Design review of the part built by this model. Coordinates are the model's own, in mm. A direction names the side the tool comes from. Give positions to 0.01 mm unless a question says otherwise; leave off trailing zeros. Order: outer loops, then holes, each group sorted by start corner. A loop starts at its lowest first (then second) coordinate and runs counter-clockwise, first axis right, second up. Notation, with made-up numbers: (59.5, 5) -> (80.5, 5) arc R24 ccw to (80.5, 38) -> close; hole circle Ø5 at (75.25, 57.25). An arc over 180 degrees is marked (long way). Answer in a Markdown table with one row per item. Add a question column.
```python
from build123d import *

# Parameters (mm, degrees)
ESQUISSE1_W              = 140
ESQUISSE1_H              = 30
BOSS_EXTRU_1_DEPTH       = 20
ESQUISSE3_W              = 140
ESQUISSE3_H              = 30
BOSS_EXTRU_2_DEPTH       = 20
BOSS_EXTRU_3_DEPTH       = 30
BOSS_EXTRU_4_DEPTH       = 30
ESQUISSE12_W             = 140
ESQUISSE12_H             = 30
ENL_V_MAT_EXTRU_1_DEPTH  = 41
ESQUISSE13_R             = 2
ENL_V_MAT_EXTRU_2_DEPTH  = 31
ESQUISSE25_R             = 2.5
ENL_V_MAT_EXTRU_11_DEPTH = 3
ENL_V_MAT_EXTRU_5_DEPTH  = 31
ENL_V_MAT_EXTRU_6_DEPTH  = 31
ESQUISSE19_W             = 12.781453569
ESQUISSE19_H             = 30
ENL_V_MAT_EXTRU_7_DEPTH  = 2
ESQUISSE20_W             = 12.289859201
ESQUISSE20_H             = 30
ENL_V_MAT_EXTRU_8_DEPTH  = 2
ENL_V_MAT_EXTRU_9_DEPTH  = 0.5
ENL_V_MAT_EXTRU_10_DEPTH = 0.5
ESQUISSE15_R             = 2.5
ENL_V_MAT_EXTRU_15_DEPTH = 3
CONG_1_R                 = 20
CONG_3_R                 = 4


with BuildPart() as part:
    # Esquisse1 → Boss.-Extru.1 (new body)
    with BuildSketch(Plane.XY):
        with Locations((70, 15)):
            Rectangle(ESQUISSE1_W, ESQUISSE1_H)
    extrude(amount=BOSS_EXTRU_1_DEPTH)

    # Esquisse3 → Boss.-Extru.2 (add)
    with BuildSketch(Plane.XY.offset(20)):
        with Locations((70, 15)):
            Rectangle(ESQUISSE3_W, ESQUISSE3_H)
    extrude(amount=BOSS_EXTRU_2_DEPTH)

    # Esquisse5 → Boss.-Extru.3 (add)
    with BuildSketch(Plane.XZ):
        Polygon((70, 12), (140, 25), (140, 12), (70, 0), align=None)
    extrude(amount=BOSS_EXTRU_3_DEPTH)

    # Esquisse6 → Boss.-Extru.4 (add)
    with BuildSketch(Plane.XZ):
        Polygon((0, 25), (0, 12.5), (70, 0), (70, 12), align=None)
    extrude(amount=BOSS_EXTRU_4_DEPTH)

    # Esquisse12 → Enlèv. mat.-Extru.1 (cut, through all)
    with BuildSketch(Plane.XY.offset(40)):
        with Locations((70, 15)):
            Rectangle(ESQUISSE12_W, ESQUISSE12_H)
    extrude(amount=-ENL_V_MAT_EXTRU_1_DEPTH, mode=Mode.SUBTRACT)

    # Esquisse13 → Enlèv. mat.-Extru.2 (cut, through all)
    with BuildSketch(Plane.XZ.offset(30)):
        with Locations((70, 6)):
            Circle(ESQUISSE13_R)
    extrude(amount=-ENL_V_MAT_EXTRU_2_DEPTH, mode=Mode.SUBTRACT)

    # Esquisse25 → Enlèv. mat.-Extru.11 (cut)
    with BuildSketch(Plane(origin=(2.1631644, 0, 12.113720643), x_dir=(-0.984427576, 0, 0.175790638), z_dir=(-0.175790638, 0, -0.984427576))):
        with Locations((-12.309930286, -15)):
            Circle(ESQUISSE25_R)
    extrude(amount=-ENL_V_MAT_EXTRU_11_DEPTH, mode=Mode.SUBTRACT)

    # Esquisse16 → Enlèv. mat.-Extru.5 (cut, through all)
    with BuildSketch(Plane(origin=(0, 0, 0), x_dir=(1, 0, 0), z_dir=(0, 1, 0))):
        Polygon((0, -12.5), (2.244032354, -24.583251134), (0, -25), align=None)
    extrude(amount=-ENL_V_MAT_EXTRU_5_DEPTH, mode=Mode.SUBTRACT)

    # Esquisse17 → Enlèv. mat.-Extru.6 (cut, through all)
    with BuildSketch(Plane(origin=(0, 0, 0), x_dir=(1, 0, 0), z_dir=(0, 1, 0))):
        Polygon((140, -12), (137.666206352, -24.56658118), (140, -25), align=None)
    extrude(amount=-ENL_V_MAT_EXTRU_6_DEPTH, mode=Mode.SUBTRACT)

    # Esquisse19 → Enlèv. mat.-Extru.7 (cut)
    with BuildSketch(Plane(origin=(137.486683764, 0, 25.53324127), x_dir=(0.182592194, 0, -0.983188736), z_dir=(0.983188736, 0, 0.182592194))):
        with Locations((7.373915521, -15)):
            Rectangle(ESQUISSE19_W, ESQUISSE19_H)
    extrude(amount=-ENL_V_MAT_EXTRU_7_DEPTH, mode=Mode.SUBTRACT)

    # Esquisse20 → Enlèv. mat.-Extru.8 (cut)
    with BuildSketch(Plane(origin=(-2.244032354, 0, 0.416748866), x_dir=(0.182592194, 0, 0.983188736), z_dir=(-0.983188736, 0, 0.182592194))):
        with Locations((18.434788802, -15)):
            Rectangle(ESQUISSE20_W, ESQUISSE20_H)
    extrude(amount=-ENL_V_MAT_EXTRU_8_DEPTH, mode=Mode.SUBTRACT)

    # Esquisse22 → Enlèv. mat.-Extru.9 (cut)
    with BuildSketch(Plane.XZ.offset(30)):
        Polygon((4.210409826, 24.218066747), (1.968902204, 12.148410321), (70, 0), (138.028566573, 11.662039984), (135.69982888, 24.201396792), (70, 12), align=None)
    extrude(amount=-ENL_V_MAT_EXTRU_9_DEPTH, mode=Mode.SUBTRACT)

    # Esquisse23 → Enlèv. mat.-Extru.10 (cut)
    with BuildSketch(Plane(origin=(0, 0, 0), x_dir=(1, 0, 0), z_dir=(0, 1, 0))):
        Polygon((1.968902204, -12.148410321), (4.210409826, -24.218066747), (70, -12), (135.69982888, -24.201396792), (138.028566573, -11.662039984), (70, 0), align=None)
    extrude(amount=-ENL_V_MAT_EXTRU_10_DEPTH, mode=Mode.SUBTRACT)

    # Esquisse15 → Enlèv. mat.-Extru.15 (cut)
    with BuildSketch(Plane(origin=(1.998413957, 0, -11.65741475), x_dir=(-0.985622255, 0, -0.168963815), z_dir=(0.168963815, 0, -0.985622255))):
        with Locations((-125.593557837, -15)):
            Circle(ESQUISSE15_R)
    extrude(amount=-ENL_V_MAT_EXTRU_15_DEPTH, mode=Mode.SUBTRACT)

    # Congé1
    cong_1_edges = [part.edges().sort_by_distance(p)[0] for p in [
        (70, -15, 12),
    ]]
    fillet(cong_1_edges, radius=CONG_1_R)

    # Congé3
    cong_3_edges = [part.edges().sort_by_distance(p)[0] for p in [
        (4.210409826, -15, 24.218066747),
        (104.675836379, -29.5, 18.439798185),
        (135.69982888, -15, 24.201396792),
        (35.279282974, -0.5, 18.448133162),
        (35.279282974, -29.5, 18.448133162),
        (104.675836379, -0.5, 18.439798185),
        (70, -0.5, 12.341974299),
        (70, -29.5, 12.341974299),
    ]]
    fillet(cong_3_edges, radius=CONG_3_R)


solid = part.part
```
1) For L1, parallel to Z at x = 70, y = -19.5; L2, parallel to Z at x = 25, y = -25.75; L3, parallel to Z at x = 75, y = -20.5, list the stretches that pass through material, from the lowest coordinate up.
2) Clearance check with flat-ended pins moving along their axes: P1, Ø3, axis at y = -5, z = 13, coming from the -X side; P2, Ø6, axis at y = -7.5, z = 19, coming from the +X side; P3, Ø4, axis at x = 25, y = -17, coming from the +Z side; P4, Ø12, axis at x = 32, y = -4, coming from the -Z side. State where each tip first meets the part, or that it passes through.
3) Machinability: for faces 1 (the face through (71.908, -15.203, 6.601)), 2 (the face through (34.636, -28.297, 17.407)), 3 (the face through (125.314, -14.965, 12.526)), 4 (the face through (37.7, -14.9, 18)), 5 (the face through (35.495, -1.641, 17.185)), which of the approach directions +Z, -Z, +X, -X, +Y, -Y give a long, thin tool a straight path to every point of the face, cutting with its end or side? Answer none if there is none.
4) Mouldability with a two-part tool opening along X and no side actions: class faces 6 (the face through (104.45, -28.297, 17.238)), 7 (the face through (14.843, -14.965, 12.897)), 8 (the face through (2.714, -14.797, 16.16)), 9 (the face through (69, -0.5, 3)) as +X half, -X half, draft (parallel to the pull), parting line (faces both ways), or undercut.
5) Add section A-A, the plane y = -19.25. Write out the cut boundary in (x, z), and give its area (3 significant figures).
6) Add section C-C, the plane y = -3. Write out the cut boundary in (x, z), and give its area (3 significant figures).
7) Add section B-B, the plane z = 6. Write out the cut boundary in (x, y).
Verdict:
| question | item | result |
|---|---|---|
| 1 | L1 | z = 0 to 4, 8 to 12.34 |
| 1 | L2 | z = 8.04 to 20.35 |
| 1 | L3 | z = 0.86 to 12.93 |
| 2 | P1 | stops at x = 1.97 |
| 2 | P2 | stops at x = 137.22 |
| 2 | P3 | stops at z = 20.73 |
| 2 | P4 | stops at z = 5.71 |
| 3 | face 1 | +Y, -Y |
| 3 | face 2 | +Z, -Y |
| 3 | face 3 | none |
| 3 | face 4 | +Z, +Y, -Y |
| 3 | face 5 | +Z, +Y |
| 4 | face 6 | undercut |
| 4 | face 7 | undercut |
| 4 | face 8 | -X half |
| 4 | face 9 | draft |
| 5 | outline | (1.97, 12.15) -> (70, 0) -> (138.03, 11.66) -> (136.43, 20.27) arc R4 ccw to (131.77, 23.47) -> (73.65, 12.68) arc R20 cw to (66.35, 12.68) -> (8.14, 23.49) arc R4 ccw to (3.48, 20.29) -> close; hole circle Ø4 at (70, 6) |
| 5 | area | 1,630 mm2 |
| 6 | outline | (1.97, 12.15) -> (70, 0) -> (138.03, 11.66) -> (136.43, 20.27) arc R4 ccw to (133.3, 23.46) -> (73.71, 12.39) arc R20.29 cw to (66.29, 12.39) -> (6.62, 23.47) arc R4 ccw to (3.48, 20.29) -> close; hole circle Ø4 at (70, 6) |
| 6 | area | 1,600 mm2 |
| 7 | outline | (36.4, -29.5) -> (68, -29.5) -> (68, -0.5) -> (36.4, -0.5) -> close; (72, -29.5) -> (105, -29.5) -> (105, -0.5) -> (72, -0.5) -> close |
